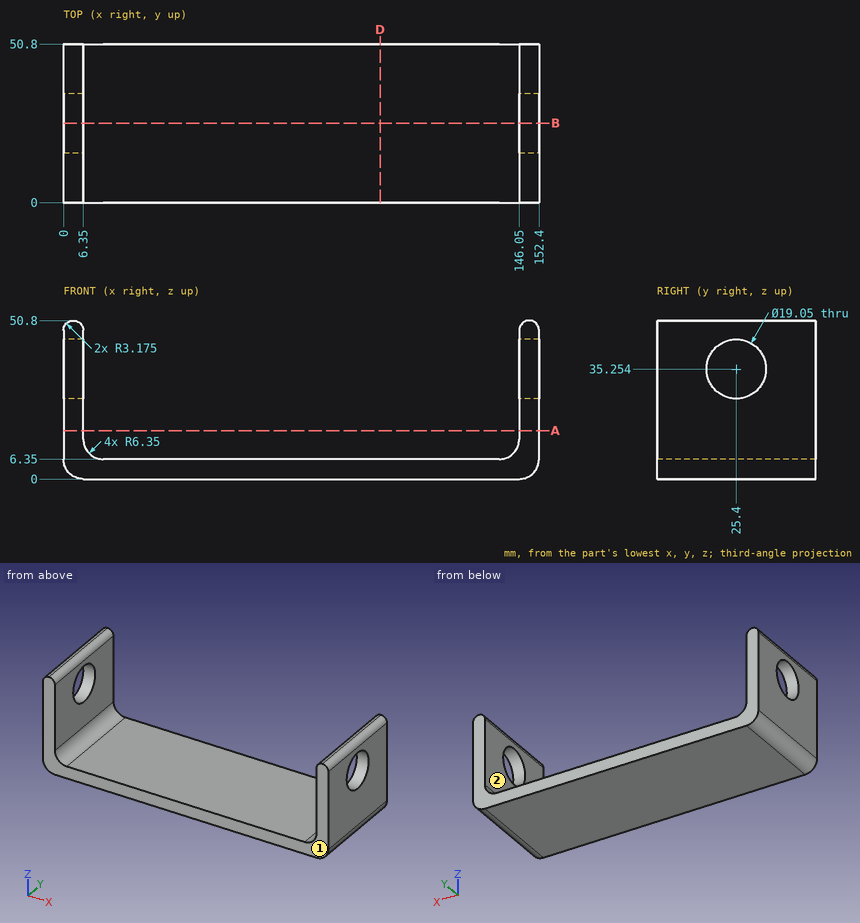
Could you check a few things on this drawing? It's one solid part, dimensions in mm from its lowest x, y, z. A direction names the side the tool comes from. Give positions to 0.01 mm unless a question says otherwise; leave off trailing zeros. Write each loop counter-clockwise with the first axis right and the second up, starting at its lowest first coordinate (ties: lowest second). Pieces come first, ordered by that corner, then holes.
(1) If I drill on L1, parallel to X at y = 34, z = 12.5; L2, parallel to Z at x = 108.5, y = 44; L3, parallel to X at y = 11, z = 11, over which ranges is the centre line in solid material (lowest first)?
Output values:
L1: x = 0 to 6.35, 146.05 to 152.4
L2: z = 0 to 6.35
L3: x = 0 to 6.58, 145.82 to 152.4
(2) Will these pins go through, and if not, where does the flat tip stop? pin 1 (12 mm diameter, centred on x = 17, y = 29, fed in from +Z); pin 2 (12 mm diameter, centred on x = 24, y = 13.5, fed in from +Z); pin 3 (4 mm diameter, centred on x = 63.5, y = 18, fed in from +Z).
Output values:
pin 1: stops at z = 6.58
pin 2: stops at z = 6.35
pin 3: stops at z = 6.35
(3) Imagine slicing it at A-A, the plane z = 15.5. Write out the boundary of the cut face in (x, y), and give its area (3 significant figures).
Output values:
outline: (0, 0) - (6.35, 0) - (6.35, 50.8) - (0, 50.8) - close; (146.05, 0) - (152.4, 0) - (152.4, 50.8) - (146.05, 50.8) - close
area: 645 mm2
(4) Imagine slicing it at B-B, the plane y = 25.4. Count the separate pieces of the cut face and the enclosed holes in it, and give its area (3 significant figures).
Output values:
separate pieces: 3
enclosed holes: 0
area: 1,280 mm2
(5) On a 3-axis mill with a long thin cutter (end or side, diameter ignored), from which of +Z, -Z, +X, -X, +Y, -Y can I reach the whole of each face in a straight line? I mean the marked faces 1 and 2. Say none if no direction works.
Output values:
face 1: +Z, -Z, +X, -X, -Y
face 2: +Z, +Y, -Y
(6) Imagine slicing it at D-D, the plane x = 101.5. Write out the boundary of the cut face in (y, z).
Output values:
outline: (0, 0) - (50.8, 0) - (50.8, 6.35) - (0, 6.35) - close
